from build123d import *

# Parameters (mm, degrees)
SKETCH1_R                    = 2
BOSS_EXTRUDE1_DEPTH          = 10
CUT_EXTRUDE2_REACH           = 24.913
SKETCH3_W                    = 8
SKETCH3_H                    = 10
BOSS_EXTRUDE2_DEPTH          = 8
F_10_5_10_5_DIAMETER_HOLE1_D = 10.5
F_3_5_3_5_DIAMETER_HOLE1_D   = 3.5
FILLET1_R                    = 1


with BuildPart() as part:
    # Sketch1 → Boss-Extrude1 (new, symmetric)
    with BuildSketch(Plane(origin=(0, 0, 0), x_dir=(1, 0, 0), z_dir=(0, 1, 0))):
        with BuildLine():
            Line((15, 4), (-15, 4))
            ThreePointArc((-15, 4), (-19, 0), (-15, -4))
            Line((-15, -4), (15, -4))
            ThreePointArc((15, -4), (19, 0), (15, 4))
        make_face()
        with Locations(Location((-15, 0, 0), (0, 0, 270))):
            Circle(SKETCH1_R, mode=Mode.SUBTRACT)
        with Locations(Location((15, 0, 0), (0, 0, 270))):
            Circle(SKETCH1_R, mode=Mode.SUBTRACT)
    extrude(amount=BOSS_EXTRUDE1_DEPTH, both=True)

    # Cut-Extrude2: up to this face of the body (flat: up to its plane)
    cut_extrude2_end = Plane(part.part.faces().sort_by_distance((0, 0, -4))[0])
    # Sketch3 → Cut-Extrude2 (cut, up to the picked face)
    with BuildSketch(Plane.XY.offset(4), mode=Mode.PRIVATE) as cut_extrude2_sk1:
        with Locations((-15, 0)):
            Rectangle(SKETCH3_W, SKETCH3_H)
    cut_extrude2_tool1 = split(extrude(cut_extrude2_sk1.sketch, amount=-CUT_EXTRUDE2_REACH, mode=Mode.PRIVATE), bisect_by=cut_extrude2_end, keep=Keep.BOTH, mode=Mode.PRIVATE)
    # Sketch3 → Cut-Extrude2 (cut, up to the picked face)
    with BuildSketch(Plane.XY.offset(4), mode=Mode.PRIVATE) as cut_extrude2_sk2:
        with Locations((15, 0)):
            Rectangle(SKETCH3_W, SKETCH3_H)
    cut_extrude2_tool2 = split(extrude(cut_extrude2_sk2.sketch, amount=-CUT_EXTRUDE2_REACH, mode=Mode.PRIVATE), bisect_by=cut_extrude2_end, keep=Keep.BOTH, mode=Mode.PRIVATE)
    add(cut_extrude2_tool1.solids().sort_by(Axis((-15, 0, 4), (0, 0, -1)))[0], mode=Mode.SUBTRACT)
    add(cut_extrude2_tool2.solids().sort_by(Axis((15, 0, 4), (0, 0, -1)))[0], mode=Mode.SUBTRACT)

    # Sketch2 → Boss-Extrude2 (add)
    with BuildSketch(Plane.XY.offset(4)):
        with BuildLine():
            Line((-5, -9.797958971), (-5, -12))
            Line((-5, -12), (5, -12))
            Line((5, -12), (5, -9.797958971))
            ThreePointArc((5, -9.797958971), (11, 0), (5, 9.797958971))
            Line((5, 9.797958971), (5, 12))
            Line((5, 12), (-5, 12))
            Line((-5, 12), (-5, 9.797958971))
            ThreePointArc((-5, 9.797958971), (-11, 0), (-5, -9.797958971))
        make_face()
    extrude(amount=-BOSS_EXTRUDE2_DEPTH)

    # Ø10.5 (10.5) Diameter Hole1 (through all)
    with Locations(Plane.XY.offset(4)):
        with Locations((0, 0)):
            Hole(F_10_5_10_5_DIAMETER_HOLE1_D / 2)

    # Ø3.5 (3.5) Diameter Hole1 (through all)
    with Locations(Plane(origin=(5.656854249, 5.656854249, 4), x_dir=(1, 0, 0), z_dir=(0, 0, 1))):
        with Locations((0, 0), (0, -11.313708498), (-11.313708498, 0), (-11.313708498, -11.313708498)):
            Hole(F_3_5_3_5_DIAMETER_HOLE1_D / 2)

    # Fillet1
    fillet1_edges = [part.edges().sort_by_distance(p)[0] for p in [
        (-5, -12, 0),
        (-5, 12, 0),
        (5, 12, 0),
        (5, -12, 0),
    ]]
    fillet(fillet1_edges, radius=FILLET1_R)


solid = part.part
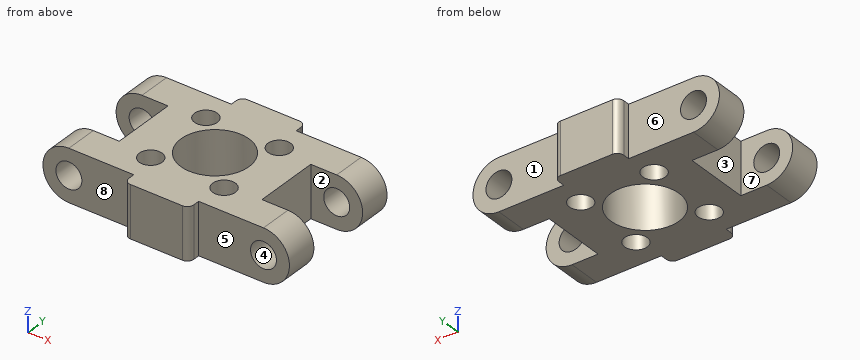
Input: part model. Units: mm. Frame: model coordinates. Face numbers are marked on the shaded views. A direction names the side the tool comes from. Round coordinates to 2 decimals unless told otherwise and drop trailing zeros. Loops run counter-clockwise (first coordinate to the right, second up) from the corner with the lowest first, then second, coordinate; pieces in that order, holes last. Notation, with made-up numbers: (83, 7) -> (130, 7) arc R20 ccw to (130, 42) -> close; hole circle Ø8 at (71.25, 19.5). An arc over 180 degrees is marked (long way). Answer as a JSON object with one key per item and string values. Group by question number.
1) Reachability of the marked faces 1, 2, 3, 4 and 5 from +Z, -Z, +X, -X, +Y, -Y: full face, straight path, thin tool, end or side. Return the list, or none.
2) Pin query (flat end, axial travel): pin 1 (1.5 mm diameter, centred on y = 6.5, z = -2, fed in from -X); pin 2 (0.8 mm diameter, centred on y = 10.5, z = 1, fed in from -X); pin 3 (0.8 mm diameter, centred on y = 10.5, z = -1.5, fed in from +X). Return the tip coordinate at first contact, or that it passes through.
3) Section query C-C on x = -6. Output: boundary loops of the cut face in (y, z).
4) Draft query along Y for the marked faces 6, 7 and 8. Return one class per face: +Y half, -Y half, draft (parallel to the pull), parting line (faces both ways), or undercut.
5) Section query B-B on x = -11.5. Output: boundary loops of the cut face in (y, z), plus the area to 3 significant figures.
6) Section query A-A on y = 0. Output: boundary loops of the cut face in (x, z).
7) Ray query, L1, parallel to X at y = -8.5, z = 0; L2, parallel to Y at x = -17, z = 0.5; L3, parallel to X at y = 4.25, z = 0.5. Return the intervals inside material, ascending.
Reply:
{
 "1": {"face 1": "+Z, -Z, +X, +Y", "face 2": "+Z, -Z, +X", "face 3": "+Z, -Z, -X", "face 4": "+Y, -Y", "face 5": "+Z, -Z, +X, -Y"},
 "2": {"pin 1": "stops at x = -18.8", "pin 2": "stops at x = -5", "pin 3": "stops at x = 5"},
 "3": {"outline": "(-10, -4) -> (-7.37, -4) -> (-7.37, 4) -> (-10, 4) -> close; (-3.94, -4) -> (3.94, -4) -> (3.94, 4) -> (-3.94, 4) -> close; (7.37, -4) -> (10, -4) -> (10, 4) -> (7.37, 4) -> close"},
 "4": {"face 6": "+Y half", "face 7": "undercut", "face 8": "-Y half"},
 "5": {"outline": "(-10, -4) -> (-5, -4) -> (-5, 4) -> (-10, 4) -> close; (5, -4) -> (10, -4) -> (10, 4) -> (5, 4) -> close", "area": "80.0 mm2"},
 "6": {"outline": "(-11, -4) -> (-5.25, -4) -> (-5.25, 4) -> (-11, 4) -> close; (5.25, -4) -> (11, -4) -> (11, 4) -> (5.25, 4) -> close"},
 "7": {"L1": "x = -19 to -17, -13 to 13, 17 to 19", "L2": "y = -10 to -5, 5 to 10", "L3": "x = -11 to -6.7, -4.62 to -3.08, 3.08 to 4.62, 6.7 to 11"}
}
